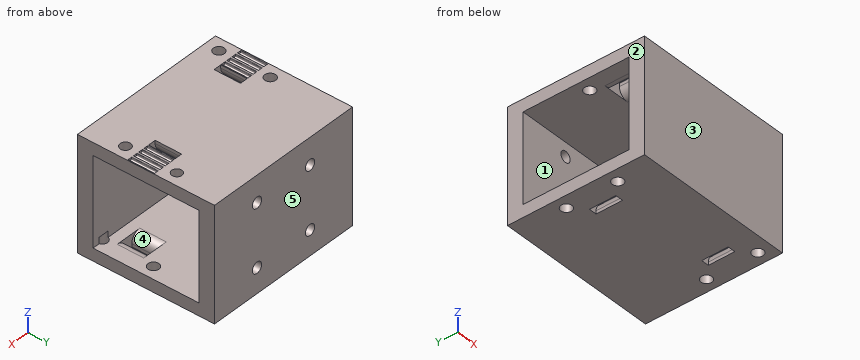
from build123d import *

# Parameters (mm, degrees)
SKETCH1_W           = 52
SKETCH1_H           = 36.5
SKETCH1_R           = 1.75
BOSS_EXTRUDE1_DEPTH = 5
SKETCH2_W           = 52
SKETCH2_H           = 4
BOSS_EXTRUDE2_DEPTH = 34
SKETCH3_W           = 52
SKETCH3_H           = 36.5
BOSS_EXTRUDE3_DEPTH = 5
SKETCH4_W           = 2.5
SKETCH4_H           = 8.5
CUT_EXTRUDE1_DEPTH  = 8
CUT_EXTRUDE2_DEPTH  = 8.5
CUT_EXTRUDE3_DEPTH  = 8.5
SKETCH7_R           = 1.75
SKETCH7_R_2         = 1.623529306
SKETCH7_R_3         = 1.694530851
CUT_EXTRUDE4_DEPTH  = 6
SKETCH8_W           = 2.5
SKETCH8_H           = 8.5
CUT_EXTRUDE5_DEPTH  = 6
FILLET1_R           = 3
SKETCH9_R           = 1.75
CUT_EXTRUDE6_DEPTH  = 6


with BuildPart() as part:
    # Sketch1 → Boss-Extrude1 (new body)
    with BuildSketch(Plane(origin=(0, 0, 0), x_dir=(1, 0, 0), z_dir=(0, 1, 0))):
        with Locations((8.063492063, 1.794973545)):
            Rectangle(SKETCH1_W, SKETCH1_H)
        with Locations((-1.936507937, 12.044973545)):
            Circle(SKETCH1_R, mode=Mode.SUBTRACT)
        with Locations((18.063492063, 12.044973545)):
            Circle(SKETCH1_R, mode=Mode.SUBTRACT)
        with Locations((18.063492063, -7.955026455)):
            Circle(SKETCH1_R, mode=Mode.SUBTRACT)
        with Locations((-1.936507937, -7.955026455)):
            Circle(SKETCH1_R, mode=Mode.SUBTRACT)
    extrude(amount=BOSS_EXTRUDE1_DEPTH)

    # Sketch2 → Boss-Extrude2 (add)
    with BuildSketch(Plane.XZ):
        with Locations((8.063492063, 14.455026455)):
            Rectangle(SKETCH2_W, SKETCH2_H)
        with Locations((8.063492063, -18.044973545)):
            Rectangle(SKETCH2_W, SKETCH2_H)
    extrude(amount=BOSS_EXTRUDE2_DEPTH)

    # Sketch3 → Boss-Extrude3 (add)
    with BuildSketch(Plane.XZ.offset(34)):
        with Locations((8.063492063, -1.794973545)):
            Rectangle(SKETCH3_W, SKETCH3_H)
    extrude(amount=BOSS_EXTRUDE3_DEPTH)

    # Sketch4 → Cut-Extrude1 (cut)
    with BuildSketch(Plane.XY.offset(16.455026455)):
        with Locations((24.813492063, -18.75)):
            Rectangle(SKETCH4_W, SKETCH4_H)
        with Locations((-8.686507937, -26.25)):
            Rectangle(SKETCH4_W, SKETCH4_H)
    extrude(amount=-CUT_EXTRUDE1_DEPTH, mode=Mode.SUBTRACT)

    # Sketch5 → Cut-Extrude2 (cut)
    with BuildSketch(Plane(origin=(0, -30.5, 0), x_dir=(1, 0, 0), z_dir=(0, 1, 0))):
        with BuildLine():
            ThreePointArc((-11.435384341, -16.016824208), (-10.936507937, -15.705026455), (-10.437631532, -16.016824208))
            ThreePointArc((-10.437631532, -16.016824208), (-10.378896222, -16.166964301), (-10.345051045, -16.324591672))
            ThreePointArc((-10.345051045, -16.324591672), (-10.295239582, -16.417797867), (-10.196332511, -16.455026455))
            Line((-10.196332511, -16.455026455), (-9.936507937, -16.455026455))
            Line((-9.936507937, -16.455026455), (-9.936507937, -17.085026455))
            Line((-9.936507937, -17.085026455), (-13.936507937, -17.085026455))
            Line((-13.936507937, -17.085026455), (-13.936507937, -16.455026455))
            Line((-13.936507937, -16.455026455), (-13.676683362, -16.455026455))
            ThreePointArc((-13.676683362, -16.455026455), (-13.577776291, -16.417797867), (-13.527964828, -16.324591672))
            ThreePointArc((-13.527964828, -16.324591672), (-13.494119651, -16.166964301), (-13.435384341, -16.016824208))
            ThreePointArc((-13.435384341, -16.016824208), (-12.936507937, -15.705026455), (-12.437631532, -16.016824208))
            ThreePointArc((-12.437631532, -16.016824208), (-12.378896222, -16.166964301), (-12.345051045, -16.324591672))
            ThreePointArc((-12.345051045, -16.324591672), (-12.295239582, -16.417797867), (-12.196332511, -16.455026455))
            Line((-12.196332511, -16.455026455), (-11.676683362, -16.455026455))
            ThreePointArc((-11.676683362, -16.455026455), (-11.577776291, -16.417797867), (-11.527964828, -16.324591672))
            ThreePointArc((-11.527964828, -16.324591672), (-11.494119651, -16.166964301), (-11.435384341, -16.016824208))
        make_face()
        with BuildLine():
            ThreePointArc((-15.435384341, -16.016824208), (-14.936507937, -15.705026455), (-14.437631532, -16.016824208))
            ThreePointArc((-14.437631532, -16.016824208), (-14.378896222, -16.166964301), (-14.345051045, -16.324591672))
            ThreePointArc((-14.345051045, -16.324591672), (-14.295239582, -16.417797867), (-14.196332511, -16.455026455))
            Line((-14.196332511, -16.455026455), (-13.936507937, -16.455026455))
            Line((-13.936507937, -16.455026455), (-13.936507937, -17.085026455))
            Line((-13.936507937, -17.085026455), (-17.936507937, -17.085026455))
            Line((-17.936507937, -17.085026455), (-17.936507937, -16.455026455))
            Line((-17.936507937, -16.455026455), (-17.676683362, -16.455026455))
            ThreePointArc((-17.676683362, -16.455026455), (-17.577776291, -16.417797867), (-17.527964828, -16.324591672))
            ThreePointArc((-17.527964828, -16.324591672), (-17.494119651, -16.166964301), (-17.435384341, -16.016824208))
            ThreePointArc((-17.435384341, -16.016824208), (-16.936507937, -15.705026455), (-16.437631532, -16.016824208))
            ThreePointArc((-16.437631532, -16.016824208), (-16.378896222, -16.166964301), (-16.345051045, -16.324591672))
            ThreePointArc((-16.345051045, -16.324591672), (-16.295239582, -16.417797867), (-16.196332511, -16.455026455))
            Line((-16.196332511, -16.455026455), (-15.676683362, -16.455026455))
            ThreePointArc((-15.676683362, -16.455026455), (-15.577776291, -16.417797867), (-15.527964828, -16.324591672))
            ThreePointArc((-15.527964828, -16.324591672), (-15.494119651, -16.166964301), (-15.435384341, -16.016824208))
        make_face()
    extrude(amount=CUT_EXTRUDE2_DEPTH, mode=Mode.SUBTRACT)

    # Sketch6 → Cut-Extrude3 (cut)
    with BuildSketch(Plane(origin=(0, -23, 0), x_dir=(1, 0, 0), z_dir=(0, 1, 0))):
        with BuildLine():
            ThreePointArc((28.564615659, -16.016824208), (29.063492063, -15.705026455), (29.562368468, -16.016824208))
            ThreePointArc((29.562368468, -16.016824208), (29.621103778, -16.166964301), (29.654948955, -16.324591672))
            ThreePointArc((29.654948955, -16.324591672), (29.704760418, -16.417797867), (29.803667489, -16.455026455))
            Line((29.803667489, -16.455026455), (30.063492063, -16.455026455))
            Line((30.063492063, -16.455026455), (30.063492063, -17.085026455))
            Line((30.063492063, -17.085026455), (26.063492063, -17.085026455))
            Line((26.063492063, -17.085026455), (26.063492063, -16.455026455))
            Line((26.063492063, -16.455026455), (26.323316638, -16.455026455))
            ThreePointArc((26.323316638, -16.455026455), (26.422223709, -16.417797867), (26.472035172, -16.324591672))
            ThreePointArc((26.472035172, -16.324591672), (26.505880349, -16.166964301), (26.564615659, -16.016824208))
            ThreePointArc((26.564615659, -16.016824208), (27.063492063, -15.705026455), (27.562368468, -16.016824208))
            ThreePointArc((27.562368468, -16.016824208), (27.621103778, -16.166964301), (27.654948955, -16.324591672))
            ThreePointArc((27.654948955, -16.324591672), (27.704760418, -16.417797867), (27.803667489, -16.455026455))
            Line((27.803667489, -16.455026455), (28.323316638, -16.455026455))
            ThreePointArc((28.323316638, -16.455026455), (28.422223709, -16.417797867), (28.472035172, -16.324591672))
            ThreePointArc((28.472035172, -16.324591672), (28.505880349, -16.166964301), (28.564615659, -16.016824208))
        make_face()
        with BuildLine():
            ThreePointArc((32.564615659, -16.016824208), (33.063492063, -15.705026455), (33.562368468, -16.016824208))
            ThreePointArc((33.562368468, -16.016824208), (33.621103778, -16.166964301), (33.654948955, -16.324591672))
            ThreePointArc((33.654948955, -16.324591672), (33.704760418, -16.417797867), (33.803667489, -16.455026455))
            Line((33.803667489, -16.455026455), (34.063492063, -16.455026455))
            Line((34.063492063, -16.455026455), (34.063492063, -17.085026455))
            Line((34.063492063, -17.085026455), (30.063492063, -17.085026455))
            Line((30.063492063, -17.085026455), (30.063492063, -16.455026455))
            Line((30.063492063, -16.455026455), (30.323316638, -16.455026455))
            ThreePointArc((30.323316638, -16.455026455), (30.422223709, -16.417797867), (30.472035172, -16.324591672))
            ThreePointArc((30.472035172, -16.324591672), (30.505880349, -16.166964301), (30.564615659, -16.016824208))
            ThreePointArc((30.564615659, -16.016824208), (31.063492063, -15.705026455), (31.562368468, -16.016824208))
            ThreePointArc((31.562368468, -16.016824208), (31.621103778, -16.166964301), (31.654948955, -16.324591672))
            ThreePointArc((31.654948955, -16.324591672), (31.704760418, -16.417797867), (31.803667489, -16.455026455))
            Line((31.803667489, -16.455026455), (32.323316638, -16.455026455))
            ThreePointArc((32.323316638, -16.455026455), (32.422223709, -16.417797867), (32.472035172, -16.324591672))
            ThreePointArc((32.472035172, -16.324591672), (32.505880349, -16.166964301), (32.564615659, -16.016824208))
        make_face()
    extrude(amount=CUT_EXTRUDE3_DEPTH, mode=Mode.SUBTRACT)

    # Sketch7 → Cut-Extrude4 (cut)
    with BuildSketch(Plane.XY.offset(16.455026455)):
        with Locations((-13.936507937, -34.5)):
            Circle(SKETCH7_R)
        with Locations((-13.936507937, -18)):
            Circle(SKETCH7_R)
        with Locations((30.063492063, -10.5)):
            Circle(SKETCH7_R_2)
        with Locations((30.063492063, -27)):
            Circle(SKETCH7_R_3)
    extrude(amount=-CUT_EXTRUDE4_DEPTH, mode=Mode.SUBTRACT)

    # Sketch8 → Cut-Extrude5 (cut)
    with BuildSketch(Plane(origin=(0, 0, -20.044973545), x_dir=(-1, 0, 0), z_dir=(0, 0, -1))):
        with Locations((-24.813492063, -26.25)):
            Rectangle(SKETCH8_W, SKETCH8_H)
        with Locations((8.686507937, -18.75)):
            Rectangle(SKETCH8_W, SKETCH8_H)
    extrude(amount=-CUT_EXTRUDE5_DEPTH, mode=Mode.SUBTRACT)

    # Fillet1
    fillet1_edges = [part.edges().sort_by_distance(p)[0] for p in [
        (-9.936507937, -18.75, -16.044973545),
        (-7.436507937, -18.75, -16.044973545),
        (23.563492063, -26.25, -16.044973545),
        (26.063492063, -26.25, -16.044973545),
        (-7.436507937, -26.25, 12.455026455),
        (-9.936507937, -26.25, 12.455026455),
        (23.563492063, -18.75, 12.455026455),
        (26.063492063, -18.75, 12.455026455),
    ]]
    fillet(fillet1_edges, radius=FILLET1_R)

    # Sketch9 → Cut-Extrude6 (cut)
    with BuildSketch(Plane(origin=(0, 0, -20.044973545), x_dir=(-1, 0, 0), z_dir=(0, 0, -1))):
        with Locations((13.936507937, -10.5)):
            Circle(SKETCH9_R)
        with Locations((13.936507937, -27)):
            Circle(SKETCH9_R)
        with Locations((-30.063492063, -18)):
            Circle(SKETCH9_R)
        with Locations((-30.063492063, -34.5)):
            Circle(SKETCH9_R)
    extrude(amount=-CUT_EXTRUDE6_DEPTH, mode=Mode.SUBTRACT)


solid = part.part
The listing builds one solid part. Answer for the finished solid, in the listing's coordinates (mm). Face numbers are marked on the shaded views. A direction names the side the tool comes from. Coordinates: 2 decimals unless noted, no trailing zeros. Order: outer loops, then holes, each group sorted by start corner. A loop starts at its lowest first (then second) coordinate and runs counter-clockwise, first axis right, second up.
Q1. Which of the six approach directions +Z, -Z, +X, -X, +Y, -Y give full straight-line access (tool end or side, diameter ignored) to the marked faces 1 and 2?
Q2. Given P1, Ø1.5, axis at y = -2, z = 6, coming from the +X side, flat-ended and moving along its own axis, determine where the tip first touches the part or whether it passes through.
Q3. Consider line 1 (Y direction, x = 20.5, z = -8); line 2 (Z direction, x = 22, y = -33); line 3 (Z direction, x = 19, y = 3). Determine where each line is inside the solid, lowest interval first.
Q4. For a pull along Y with two mould halves and no side action, classify the marked faces 3, 4 and 5 as pulls with the +Y half, pulls with the -Y half, needs draft (parallel to the pull), parting line crosses it, or undercut.
Q5. A cutting plane is placed at B-B, the plane y = -10.5. Write down the section's boundary in (x, z), and give its area (3 significant figures).
Q6. A cutting plane is placed at D-D, the plane y = -27. State how many separate pieces and enclosed holes the cut face has, and give its area (3 significant figures).
Q7. A cutting plane is placed at A-A, the plane x = 13.5. Write down the section's boundary in (y, z).
Q8. A cutting plane is placed at C-C, the plane z = -2.5. Write down the section's boundary in (x, y), and give its area (3 significant figures).
Answers follow:
1. face 1: +X, -X
1. face 2: +Z, -Z, -X, +Y, -Y
2. P1: passes through
3. line 1: y = -39 to -34, 0 to 5
3. line 2: z = -20.04 to -16.04, 12.46 to 16.46
3. line 3: z = -20.04 to -13.52, -10.57 to 6.48, 9.43 to 16.46
4. face 3: pulls with the -Y half
4. face 4: undercut
4. face 5: pulls with the +Y half
5. outline: (-17.94, -20.04) - (-15.69, -20.04) - (-15.69, -16.04) - (-17.94, -16.04) - close; (-17.94, 12.46) - (28.44, 12.46) - (28.44, 16.46) - (-17.94, 16.46) - close; (-12.19, -20.04) - (34.06, -20.04) - (34.06, -16.04) - (-12.19, -16.04) - close; (31.69, 12.46) - (34.06, 12.46) - (34.06, 16.46) - (31.69, 16.46) - close
5. area: 389 mm2
6. separate pieces: 6
6. enclosed holes: 0
6. area: 358 mm2
7. outline: (-39, -20.04) - (5, -20.04) - (5, 16.46) - (-39, 16.46) - close; hole (-34, -16.04) - (0, -16.04) - (0, 12.46) - (-34, 12.46) - close
8. outline: (-17.94, -39) - (34.06, -39) - (34.06, -34) - (-17.94, -34) - close; (-17.94, 0) - (34.06, 0) - (34.06, 5) - (-17.94, 5) - close
8. area: 520 mm2
